Read the model definition and answer for the solid it produces. Units are mm, in the model's axes. Face numbers are marked on the shaded views. A direction names the side the tool comes from. Round coordinates to 2 decimals unless told otherwise and drop trailing zeros. Write each loop counter-clockwise with the first axis right and the second up, starting at its lowest first coordinate (ties: lowest second). Pieces come first, ordered by that corner, then holes.
from build123d import *

# Parameters (mm, degrees)
SKETCH2_R           = 1.4986
BOSS_EXTRUDE3_DEPTH = 3.175
BOSS_EXTRUDE4_DEPTH = 25.4
SKETCH8_R           = 4.699
SKETCH8_R_2         = 1.524
BOSS_EXTRUDE5_DEPTH = 6.35
SKETCH8_3_R         = 1.524
CUT_EXTRUDE1_DEPTH  = 4.175
SKETCH10_R          = 3.556
SKETCH10_R_2        = 1.016
SKETCH10_R_3        = 4.699
SKETCH10_R_4        = 4.445
BOSS_EXTRUDE6_DEPTH = 3.175
SKETCH10_2_R        = 1.016
CUT_EXTRUDE2_DEPTH  = 4.175
SKETCH11_R          = 2.54
SKETCH11_R_2        = 1.016
BOSS_EXTRUDE7_DEPTH = 12.7
SKETCH11_2_R        = 1.016
CUT_EXTRUDE3_DEPTH  = 4.175
SKETCH12_W          = 25.4
SKETCH12_H          = 25.4
BOSS_EXTRUDE8_DEPTH = 25.4
SKETCH13_R          = 3.175
CUT_EXTRUDE4_DEPTH  = 157.21
SKETCH14_R          = 3.175
SKETCH14_R_2        = 1.524
BOSS_EXTRUDE9_DEPTH = 3.175
SKETCH16_R          = 1.524
CUT_EXTRUDE5_DEPTH  = 4.175


with BuildPart() as part:
    # Sketch2 → Boss-Extrude3 (new body)
    with BuildSketch(Plane(origin=(0, 0, 0), x_dir=(1, 0, 0), z_dir=(0, 1, 0))):
        Polygon((-61.101730223, 40.053150292), (88.758269777, 40.053150292), (91.933269777, 40.053150292), (91.933269777, -232.996849708), (88.758269777, -232.996849708), (-61.101730223, -232.996849708), (-64.276730223, -232.996849708), (-64.276730223, 40.053150292), align=None)
        with Locations((-56.339230223, -182.196849708)):
            Circle(SKETCH2_R, mode=Mode.SUBTRACT)
        with Locations((83.995769777, -182.196849708)):
            Circle(SKETCH2_R, mode=Mode.SUBTRACT)
        with Locations((-56.339230223, -29.796849708)):
            Circle(SKETCH2_R, mode=Mode.SUBTRACT)
        with Locations((83.995769777, -29.796849708)):
            Circle(SKETCH2_R, mode=Mode.SUBTRACT)
    extrude(amount=BOSS_EXTRUDE3_DEPTH)

    # Sketch7 → Boss-Extrude4 (add)
    with BuildSketch(Plane(origin=(0, 3.175, 0), x_dir=(1, 0, 0), z_dir=(0, 1, 0))):
        Polygon((-35.701730223, 40.053150292), (-64.276730223, 40.053150292), (-64.276730223, -232.996849708), (91.933269777, -232.996849708), (91.933269777, 40.053150292), (63.358269777, 40.053150292), (63.358269777, 36.878150292), (88.758269777, 36.878150292), (88.758269777, -229.821849708), (-61.101730223, -229.821849708), (-61.101730223, 36.878150292), (-35.701730223, 36.878150292), align=None)
    extrude(amount=BOSS_EXTRUDE4_DEPTH)

    # Sketch8 → Boss-Extrude5 (add)
    with BuildSketch(Plane(origin=(0, 3.175, 0), x_dir=(1, 0, 0), z_dir=(0, 1, 0))):
        with Locations((-4.840730223, 30.020150292)):
            Circle(SKETCH8_R)
        with Locations((-4.840730223, 30.020150292)):
            Circle(SKETCH8_R_2, mode=Mode.SUBTRACT)
        with Locations((-19.699730223, -22.176849708)):
            Circle(SKETCH8_R)
        with Locations((-19.699730223, -22.176849708)):
            Circle(SKETCH8_R_2, mode=Mode.SUBTRACT)
        with Locations((44.562269777, 7.541150292)):
            Circle(SKETCH8_R)
        with Locations((44.562269777, 7.541150292)):
            Circle(SKETCH8_R_2, mode=Mode.SUBTRACT)
        with Locations((46.213269777, -36.019849708)):
            Circle(SKETCH8_R)
        with Locations((46.213269777, -36.019849708)):
            Circle(SKETCH8_R_2, mode=Mode.SUBTRACT)
    extrude(amount=BOSS_EXTRUDE5_DEPTH)

    # Sketch8_3 → Cut-Extrude1 (cut, through all)
    with BuildSketch(Plane(origin=(0, 3.175, 0), x_dir=(1, 0, 0), z_dir=(0, 1, 0))):
        with Locations((-4.840730223, 30.020150292)):
            Circle(SKETCH8_3_R)
        with Locations((44.562269777, 7.541150292)):
            Circle(SKETCH8_3_R)
        with Locations((-19.699730223, -22.176849708)):
            Circle(SKETCH8_3_R)
        with Locations((46.213269777, -36.019849708)):
            Circle(SKETCH8_3_R)
    extrude(amount=-CUT_EXTRUDE1_DEPTH, mode=Mode.SUBTRACT)

    # Sketch10 → Boss-Extrude6 (add)
    with BuildSketch(Plane(origin=(0, 3.175, 0), x_dir=(1, 0, 0), z_dir=(0, 1, 0))):
        with Locations((-56.339230223, -67.896849708)):
            Circle(SKETCH10_R)
        with Locations((-56.339230223, -67.896849708)):
            Circle(SKETCH10_R_2, mode=Mode.SUBTRACT)
        with Locations((-35.041330223, -67.896849708)):
            Circle(SKETCH10_R_3)
        with Locations((-35.041330223, -67.896849708)):
            Circle(SKETCH10_R_2, mode=Mode.SUBTRACT)
        with Locations((-56.339230223, -123.192649708)):
            Circle(SKETCH10_R)
        with Locations((-56.339230223, -123.192649708)):
            Circle(SKETCH10_R_2, mode=Mode.SUBTRACT)
        with Locations((-35.041330223, -123.192649708)):
            Circle(SKETCH10_R_3)
        with Locations((-35.041330223, -123.192649708)):
            Circle(SKETCH10_R_2, mode=Mode.SUBTRACT)
        with Locations((-0.292403635, -50.864423121)):
            Circle(SKETCH10_R_4)
        with Locations((-0.292403635, -50.864423121)):
            Circle(SKETCH10_R_2, mode=Mode.SUBTRACT)
        with Locations((23.151796365, -50.864423121)):
            Circle(SKETCH10_R_4)
        with Locations((23.151796365, -50.864423121)):
            Circle(SKETCH10_R_2, mode=Mode.SUBTRACT)
        with Locations((23.151796365, -73.851423121)):
            Circle(SKETCH10_R_4)
        with Locations((23.151796365, -73.851423121)):
            Circle(SKETCH10_R_2, mode=Mode.SUBTRACT)
        with Locations((-0.292403635, -73.851423121)):
            Circle(SKETCH10_R_4)
        with Locations((-0.292403635, -73.851423121)):
            Circle(SKETCH10_R_2, mode=Mode.SUBTRACT)
    extrude(amount=BOSS_EXTRUDE6_DEPTH)

    # Sketch10_2 → Cut-Extrude2 (cut, through all)
    with BuildSketch(Plane(origin=(0, 3.175, 0), x_dir=(1, 0, 0), z_dir=(0, 1, 0))):
        with Locations((-56.339230223, -67.896849708)):
            Circle(SKETCH10_2_R)
        with Locations((-35.041330223, -67.896849708)):
            Circle(SKETCH10_2_R)
        with Locations((-35.041330223, -123.192649708)):
            Circle(SKETCH10_2_R)
        with Locations((-56.339230223, -123.192649708)):
            Circle(SKETCH10_2_R)
        with Locations((-0.292403635, -50.864423121)):
            Circle(SKETCH10_2_R)
        with Locations((23.151796365, -50.864423121)):
            Circle(SKETCH10_2_R)
        with Locations((-0.292403635, -73.851423121)):
            Circle(SKETCH10_2_R)
        with Locations((23.151796365, -73.851423121)):
            Circle(SKETCH10_2_R)
    extrude(amount=-CUT_EXTRUDE2_DEPTH, mode=Mode.SUBTRACT)

    # Sketch11 → Boss-Extrude7 (add)
    with BuildSketch(Plane(origin=(0, 3.175, 0), x_dir=(1, 0, 0), z_dir=(0, 1, 0))):
        with Locations((-27.287980223, -223.802049708)):
            Circle(SKETCH11_R)
        with Locations((-27.287980223, -223.802049708)):
            Circle(SKETCH11_R_2, mode=Mode.SUBTRACT)
        with Locations((-27.311451073, -165.890049708)):
            Circle(SKETCH11_R)
        with Locations((-27.311451073, -165.890049708)):
            Circle(SKETCH11_R_2, mode=Mode.SUBTRACT)
        with Locations((58.691019777, -165.890049708)):
            Circle(SKETCH11_R)
        with Locations((58.691019777, -165.890049708)):
            Circle(SKETCH11_R_2, mode=Mode.SUBTRACT)
        with Locations((58.691019777, -223.802049708)):
            Circle(SKETCH11_R)
        with Locations((58.691019777, -223.802049708)):
            Circle(SKETCH11_R_2, mode=Mode.SUBTRACT)
    extrude(amount=BOSS_EXTRUDE7_DEPTH)

    # Sketch11_2 → Cut-Extrude3 (cut, through all)
    with BuildSketch(Plane(origin=(0, 3.175, 0), x_dir=(1, 0, 0), z_dir=(0, 1, 0))):
        with Locations((-27.311451073, -165.890049708)):
            Circle(SKETCH11_2_R)
        with Locations((58.691019777, -165.890049708)):
            Circle(SKETCH11_2_R)
        with Locations((58.691019777, -223.802049708)):
            Circle(SKETCH11_2_R)
        with Locations((-27.287980223, -223.802049708)):
            Circle(SKETCH11_2_R)
    extrude(amount=-CUT_EXTRUDE3_DEPTH, mode=Mode.SUBTRACT)

    # Sketch12 → Boss-Extrude8 (add)
    with BuildSketch(Plane(origin=(0, 3.175, 0), x_dir=(1, 0, 0), z_dir=(0, 1, 0))):
        with Locations((76.058269777, 24.178150292)):
            Rectangle(SKETCH12_W, SKETCH12_H)
        with Locations((-48.401730223, 24.178150292)):
            Rectangle(SKETCH12_W, SKETCH12_H)
    extrude(amount=BOSS_EXTRUDE8_DEPTH)

    # Sketch13 → Cut-Extrude4 (cut, through all)
    with BuildSketch(Plane.ZY.offset(64.276730223)):
        with Locations((201.246849708, 14.2875)):
            Circle(SKETCH13_R)
    extrude(amount=-CUT_EXTRUDE4_DEPTH, mode=Mode.SUBTRACT)

    # Sketch14 → Boss-Extrude9 (add)
    with BuildSketch(Plane(origin=(0, 3.175, 0), x_dir=(1, 0, 0), z_dir=(0, 1, 0))):
        with Locations((-0.978203635, -83.376423121)):
            Circle(SKETCH14_R)
        with Locations((-0.978203635, -83.376423121)):
            Circle(SKETCH14_R_2, mode=Mode.SUBTRACT)
        with Locations((-0.978203635, -107.506423121)):
            Circle(SKETCH14_R)
        with Locations((-0.978203635, -107.506423121)):
            Circle(SKETCH14_R_2, mode=Mode.SUBTRACT)
        with Locations((23.151796365, -83.376423121)):
            Circle(SKETCH14_R)
        with Locations((23.151796365, -83.376423121)):
            Circle(SKETCH14_R_2, mode=Mode.SUBTRACT)
        with Locations((23.151796365, -107.506423121)):
            Circle(SKETCH14_R)
        with Locations((23.151796365, -107.506423121)):
            Circle(SKETCH14_R_2, mode=Mode.SUBTRACT)
    extrude(amount=BOSS_EXTRUDE9_DEPTH)

    # Sketch16 → Cut-Extrude5 (cut, through all)
    with BuildSketch(Plane(origin=(0, 3.175, 0), x_dir=(1, 0, 0), z_dir=(0, 1, 0))):
        with Locations((-0.978203635, -83.376423121)):
            Circle(SKETCH16_R)
        with Locations((23.151796365, -83.376423121)):
            Circle(SKETCH16_R)
        with Locations((23.151796365, -107.506423121)):
            Circle(SKETCH16_R)
        with Locations((-0.978203635, -107.506423121)):
            Circle(SKETCH16_R)
    extrude(amount=-CUT_EXTRUDE5_DEPTH, mode=Mode.SUBTRACT)


solid = part.part
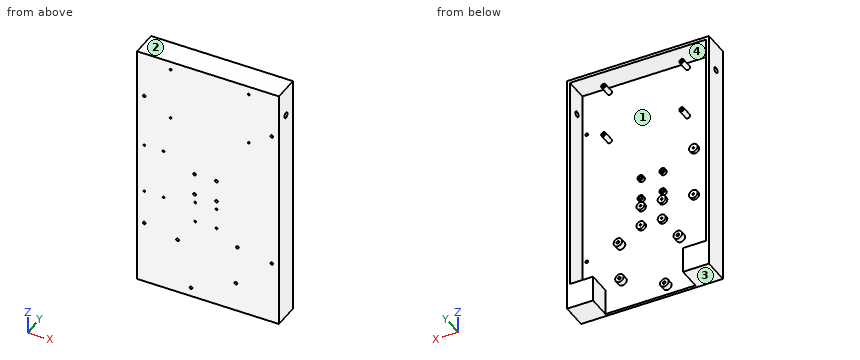
Q1. Flat-ended cylindrical pins translate along their axes: pin 1 Ø7.5 at (x, z) = (-35.5, 124.5) entering from +Y; pin 2 Ø3 at (x, z) = (71, 168) entering from -Y; pin 3 Ø3 at (x, z) = (-6, -28) entering from +Y (3 decimals). Find the tip coordinate at first contact, or state that the pin passes through.
Verdict:
pin 1: stops at y = 6.35
pin 2: stops at y = 0
pin 3: stops at y = 9.525
Q2. Which of the six approach directions +Z, -Z, +X, -X, +Y, -Y give full straight-line access (tool end or side, diameter ignored) to the marked faces 1 and 2?
Verdict:
face 1: +Y
face 2: +Z, +X, -X, +Y, -Y
Q3. Section B-B (x = -47) is taken. Determine the outline of the cut face in (y, z) (3 decimals), then the cut area to 3 significant figures.
Verdict:
outline: (0, -40.053) - (28.575, -40.053) - (28.575, -11.478) - (3.175, -11.478) - (3.175, 229.822) - (28.575, 229.822) - (28.575, 232.997) - (0, 232.997) - close
area: 1,670 mm2
Q4. Straight lines are drawn through the part: probe 1 along X at (y, z) = (15.25, 158.5); probe 2 along Z at (x, y) = (-48.5, 8.5); probe 3 along Z at (x, y) = (21, 3.75). For each, find the intervals that lie inside material, in ascending order.
Verdict:
probe 1: x = -64.28 to -61.1, 88.76 to 91.93
probe 2: z = -40.05 to -11.48, 229.82 to 233
probe 3: z = 46.97 to 54.75, 69.96 to 77.74, 81.04 to 85.71, 105.17 to 109.84, 229.82 to 233
Q5. Section A-A (z = -15) is taken. Determine the outline of the cut face in (x, y) (3 decimals).
Verdict:
outline: (-64.277, 0) - (91.933, 0) - (91.933, 28.575) - (63.358, 28.575) - (63.358, 3.175) - (-35.702, 3.175) - (-35.702, 28.575) - (-64.277, 28.575) - close
Q6. Determine the mould class of the marked faces 3 and 4 for opening direction X: pulls with the +X half, pulls with the -X half, needs draft (parallel to the pull), parting line crosses it, or undercut.
Verdict:
face 3: needs draft
face 4: undercut
